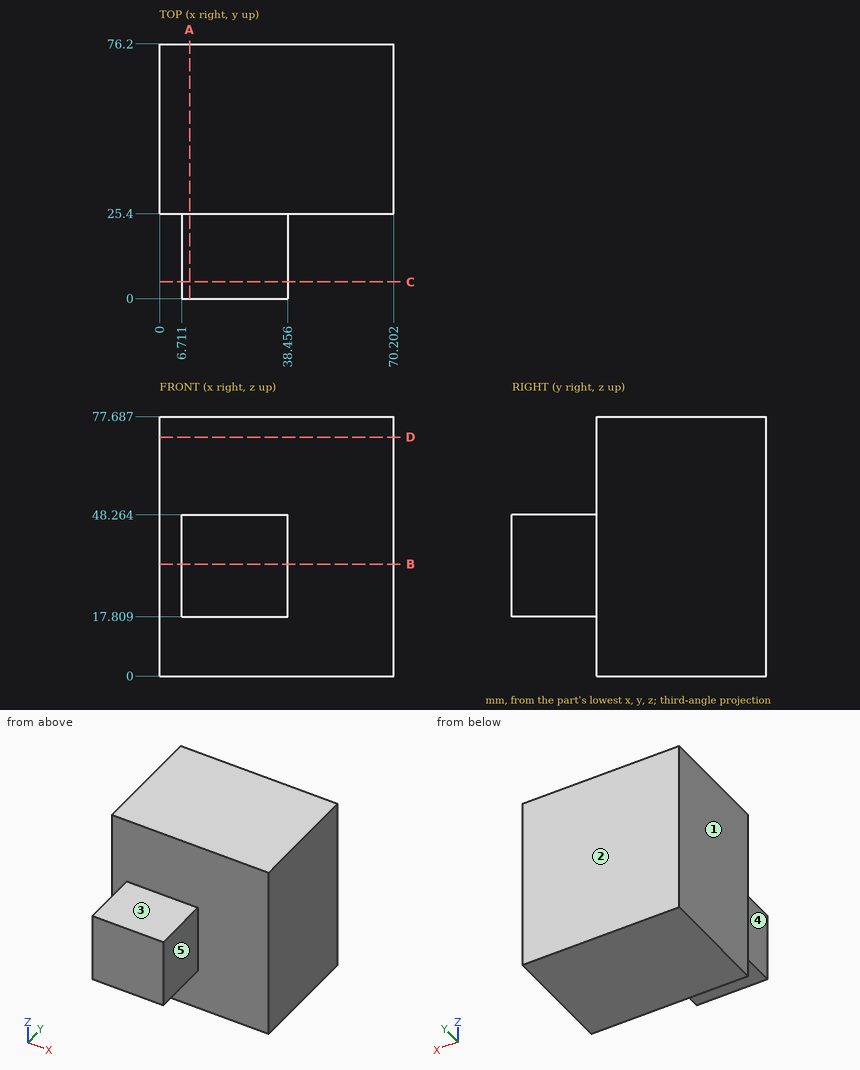
Part print with two shaded views. Sizes in mm from the minimum x, y, z corner. A direction names the side the tool comes from. Round coordinates to 2 decimals unless told otherwise and drop trailing zeros. Order: outer loops, then holes, each group sorted by start corner. A loop starts at its lowest first (then second) coordinate and runs counter-clockwise, first axis right, second up. Notation, with made-up numbers: (-37.75, -23.5) -> (14.25, -23.5) arc R21 ccw to (14.25, 2.5) -> close; hole circle Ø4 at (38.5, -1). An arc over 180 degrees is marked (long way). One line per question, with ' | ' between items.
Q1. Slice it at B-B (z = 33.5). Write the cut outline in (x, y), then the cut area to 3 significant figures.
Completed:
outline: (0, 25.4) -> (6.71, 25.4) -> (6.71, 0) -> (38.46, 0) -> (38.46, 25.4) -> (70.2, 25.4) -> (70.2, 76.2) -> (0, 76.2) -> close | area: 4,370 mm^2
Q2. Slice it at A-A (x = 9). Write the cut outline in (y, z) (1 decimal), then the cut area to 3 significant figures.
Completed:
outline: (0, 17.8) -> (25.4, 17.8) -> (25.4, 0) -> (76.2, 0) -> (76.2, 77.7) -> (25.4, 77.7) -> (25.4, 48.3) -> (0, 48.3) -> close | area: 4,720 mm^2
Q3. Slice it at C-C (y = 5). Write the cut outline in (x, z) (1 decimal).
Completed:
outline: (6.7, 17.8) -> (38.5, 17.8) -> (38.5, 48.3) -> (6.7, 48.3) -> close
Q4. Probe probe 1 along Y at (x, z) = (46, 5); probe 2 along Z at (x, y) = (11, 22.5) (1 decimal); probe 3 along X at (y, z) = (19.5, 44.5). List the from-to ranges inside material, lowest first.
Completed:
probe 1: y = 25.4 to 76.2 | probe 2: z = 17.8 to 48.3 | probe 3: x = 6.71 to 38.46
Q5. Which spindle directions (+Z, -Z, +X, -X, +Y, -Y) get a long thin tool onto all of the face, cutting with end or side? Do the marked faces 1, 2, 3, 4 and 5. Say none if no direction does.
Completed:
face 1: +Z, -Z, -X, +Y, -Y | face 2: +Z, -Z, +X, -X, +Y | face 3: +Z, +X, -X, -Y | face 4: +Z, -Z, -X, -Y | face 5: +Z, -Z, +X, -Y
Q6. Slice it at D-D (z = 71.5). Write the cut outline in (x, y), then the cut area to 3 significant figures.
Completed:
outline: (0, 25.4) -> (70.2, 25.4) -> (70.2, 76.2) -> (0, 76.2) -> close | area: 3,570 mm^2
Q7. Drop flat-ended pins along their axis: pin 1 (12.5 mm diameter, centred on x = 25.5, y = 8.5, fed in from -Z); pin 2 (1.5 mm diameter, centred on x = 10, y = 18.5, fed in from +Z); pin 3 (20.5 mm diameter, centred on y = 10, z = 34, fed in from -X). Give the stop position or say it passes through.
Completed:
pin 1: stops at z = 17.81 | pin 2: stops at z = 48.26 | pin 3: stops at x = 6.71
